Read the model definition and answer for the solid it produces. Units are mm, in the model's axes. Face numbers are marked on the shaded views. A direction names the side the tool comes from. Give positions to 0.01 mm unless a question says otherwise; leave off trailing zeros. Write each loop counter-clockwise with the first axis right and the second up, starting at its lowest first coordinate (ties: lowest second). Pieces come first, ordered by that corner, then holes. Notation, with made-up numbers: M 16,63 L 67,63 A23 cw 67,95 Z; hole C 50,12 d10. An arc over 180 degrees is marked long. Put each result on its own line as item: value.
Autodesk Inventor part; units mm, degrees
ref_plane "YZ Plane" through (0, 0, 0) normal (1, 0, 0) x (0, 1, 0)
ref_plane "XZ Plane" through (0, 0, 0) normal (0, 1, 0) x (-1, 0, 0)
ref_plane "XY Plane" through (0, 0, 0) normal (0, 0, 1) x (1, 0, 0)
sketch "Sketch_1" plane through (0, 0, 0) normal (0, 0, 1) x (1, 0, 0)
  line L0 (0, 28.85) -> (0, 9.95)
  line L1 (0, 9.95) -> (15, 9.95)
  line L2 (15, 9.95) -> (15, 28.85)
  arc A0 (15, 28.85) -> (14, 29.85) centre (14, 28.85) ccw
  line L3 (14, 29.85) -> (1, 29.85)
  arc A1 (1, 29.85) -> (0, 28.85) centre (1, 28.85) ccw
extrude "Extrusion1" add sketch "Sketch_1" against normal blind 30
sketch "Sketch_6" plane through (7.5, 0, 0) normal (1, 0, 0) x (0, 0, -1)
  line L0 (0, 21.4) -> (35, 21.4)
  line L1 (35, 21.4) -> (35, 18.15)
  line L2 (35, 18.15) -> (34.5, 18.65)
  line L3 (34.5, 18.65) -> (0.5, 18.65)
  line L4 (0.5, 18.65) -> (0, 18.15)
  line L5 (0, 18.15) -> (0, 21.4)
  line L6 (0, 21.4) -> (35, 21.4)
revolve "Revolution1" cut sketch "Sketch_6" angle 360 about axis through (7.5, 21.4, 0) along (0, 0, 1)
sketch "Sketch_4" plane through (7.5, 0, 0) normal (1, 0, 0) x (0, 0, -1)
  line L0 (0, 22.5) -> (35, 22.5)
  line L1 (35, 22.5) -> (35, 19.25)
  line L2 (35, 19.25) -> (34.5, 19.75)
  line L3 (34.5, 19.75) -> (0.5, 19.75)
  line L4 (0.5, 19.75) -> (0, 19.25)
  line L5 (0, 19.25) -> (0, 22.5)
  line L6 (0, 22.5) -> (35, 22.5)
revolve "Revolution2" cut sketch "Sketch_4" angle 360 about axis through (7.5, 22.5, 0) along (0, 0, 1)
sketch "Sketch_8" plane through (0, 21.95, 0) normal (0, 1, 0) x (1, 0, 0)
  line L0 (4.25, 0) -> (10.75, 0)
  line L1 (10.75, 0) -> (10.25, 0.5)
  line L2 (10.25, 0.5) -> (10.25, 34.5)
  line L3 (10.25, 34.5) -> (10.75, 35)
  line L4 (10.75, 35) -> (4.25, 35)
  line L5 (4.25, 35) -> (4.75, 34.5)
  line L6 (4.75, 34.5) -> (4.75, 0.5)
  line L7 (4.75, 0.5) -> (4.25, 0)
extrude "Extrusion2" cut sketch "Sketch_8" along normal mid plane 1.1
sketch "Sketch_10" plane through (0, 0, -0.5) normal (0, 0, 1) x (1, 0, 0)
  arc A0 (4.75, 21.4) -> (10.25, 21.4) centre (7.5, 21.4) ccw
  line L0 (10.25, 21.4) -> (10.25, 22.5)
  arc A1 (10.25, 22.5) -> (4.75, 22.5) centre (7.5, 22.5) ccw
  line L1 (4.75, 22.5) -> (4.75, 21.4)
extrude "Extrusion3" add sketch "Sketch_10" against normal blind 29
sketch "Sketch_11" plane through (7.5, 0, 0) normal (1, 0, 0) x (0, 0, -1)
  line L0 (0.5, 21.95) -> (29.5, 21.95)
  line L1 (29.5, 21.95) -> (29.5, 19.45)
  line L2 (29.5, 19.45) -> (29.067, 19.883)
  line L3 (29.067, 19.883) -> (0.933, 19.883)
  line L4 (0.933, 19.883) -> (0.5, 19.45)
  line L5 (0.5, 19.45) -> (0.5, 21.95)
  line L6 (0.5, 21.95) -> (29.5, 21.95)
revolve "Revolution3" cut sketch "Sketch_11" angle 360 about axis through (7.5, 21.95, -0.5) along (0, 0, 1)
thread "Thread1"
sketch "_____2" plane through (0, 9.95, 0) normal (0, 1, 0) x (1, 0, 0)
  line L0 (2.75, 17.75) -> (2.75, 14.75)
  arc A0 (2.75, 14.75) -> (7.25, 10.25) centre (7.25, 14.75) ccw
  line L1 (7.25, 10.25) -> (10.25, 10.25)
  arc A1 (10.25, 10.25) -> (12.25, 12.25) centre (10.25, 12.25) ccw
  line L2 (12.25, 12.25) -> (12.25, 15.25)
  arc A2 (12.25, 15.25) -> (7.75, 19.75) centre (7.75, 15.25) ccw
  line L3 (7.75, 19.75) -> (4.75, 19.75)
  arc A3 (4.75, 19.75) -> (2.75, 17.75) centre (4.75, 17.75) ccw
extrude "Extrusion4" add sketch "_____2" against normal blind 9.6
sketch "_____3" plane through (7.5, 0, 0) normal (1, 0, 0) x (0, 0, -1)
  line L0 (5.5, 4.65) -> (5.5, 2.35)
  arc A0 (5.5, 2.35) -> (7.5, 0.35) centre (7.5, 2.35) ccw
  line L1 (7.5, 0.35) -> (22.5, 0.35)
  arc A1 (22.5, 0.35) -> (24.5, 2.35) centre (22.5, 2.35) ccw
  line L2 (24.5, 2.35) -> (24.5, 4.65)
  line L3 (24.5, 4.65) -> (5.5, 4.65)
extrude "Extrusion5" add sketch "_____3" along normal mid plane 9.5
sketch "_____4" plane through (0, 0, -14.75) normal (0, 0, 1) x (1, 0, 0)
  line L0 (2.75, 4.25) -> (7.5, 4.65)
  line L1 (7.5, 4.65) -> (2.75, 4.65)
  line L2 (2.75, 4.65) -> (2.75, 4.25)
extrude "Extrusion6" cut sketch "_____4" along normal blind 9.5
sketch "_____5" plane through (0, 0, -15.25) normal (0, 0, 1) x (1, 0, 0)
  line L0 (7.5, 4.65) -> (12.25, 4.25)
  line L1 (12.25, 4.25) -> (12.25, 4.65)
  line L2 (12.25, 4.65) -> (7.5, 4.65)
extrude "Extrusion7" cut sketch "_____5" against normal blind 9.5
sketch "_____7" plane through (0, 0.35, 0) normal (0, 1, 0) x (1, 0, 0)
  line L0 (2.75, 17.75) -> (2.75, 14.75)
  arc A0 (2.75, 14.75) -> (7.25, 10.25) centre (7.25, 14.75) ccw
  line L1 (7.25, 10.25) -> (10.25, 10.25)
  arc A1 (10.25, 10.25) -> (12.25, 12.25) centre (10.25, 12.25) ccw
  line L2 (12.25, 12.25) -> (12.25, 15.25)
  arc A2 (12.25, 15.25) -> (7.75, 19.75) centre (7.75, 15.25) ccw
  line L3 (7.75, 19.75) -> (4.75, 19.75)
  arc A3 (4.75, 19.75) -> (2.75, 17.75) centre (4.75, 17.75) ccw
extrude "Extrusion8" add sketch "_____7" along normal blind 4.3
sketch "_____1" plane through (0, 0.35, 0) normal (0, 1, 0) x (1, 0, 0)
  line L0 (-10.5888, -9.9588) -> (25.3573, -9.9588)
  line L1 (25.3573, -9.9588) -> (25.3573, 39.1524)
  line L2 (25.3573, 39.1524) -> (-10.5888, 39.1524)
  line L3 (-10.5888, 39.1524) -> (-10.5888, -9.9588)
  arc A0 (2.75, 10.3) -> (7.55, 5.5) centre (7.55, 10.3) ccw
  line L4 (7.55, 5.5) -> (12.25, 5.5)
  line L5 (12.25, 5.5) -> (12.25, 19.7)
  arc A1 (12.25, 19.7) -> (7.45, 24.5) centre (7.45, 19.7) ccw
  line L6 (7.45, 24.5) -> (2.75, 24.5)
  line L7 (2.75, 24.5) -> (2.75, 10.3)
extrude "Extrusion9" cut sketch "_____1" along normal mid plane 19.2
sketch "Sketch_3" plane through (7.5, 0, 0) normal (1, 0, 0) x (0, 0, -1)
  line L0 (15, 0.35) -> (15, -1.45)
  line L1 (15, -1.45) -> (14.5, -1.45)
  line L2 (14.5, -1.45) -> (13, 0.35)
  line L3 (13, 0.35) -> (15, 0.35)
  line L4 (15, 0.35) -> (15, -1.45)
revolve "Revolution4" add sketch "Sketch_3" angle 360 about axis through (7.5, 0.35, -15) along (0, 1, 0)
sketch "Sketch_7" plane through (15, 0, 0) normal (1, 0, 0) x (0, 0, -1)
  line L0 (2, 15.2) -> (2, 11.95)
  line L1 (2, 11.95) -> (14, 11.95)
  line L2 (14, 11.95) -> (14, 15.2)
  line L3 (14, 15.2) -> (2, 15.2)
extrude "Extrusion10" cut sketch "Sketch_7" against normal blind 15
sketch "Sketch_5" plane through (15, 0, 0) normal (1, 0, 0) x (0, 0, -1)
  line L0 (16, 15.2) -> (16, 11.95)
  line L1 (16, 11.95) -> (28, 11.95)
  line L2 (28, 11.95) -> (28, 15.2)
  line L3 (28, 15.2) -> (16, 15.2)
extrude "Extrusion11" cut sketch "Sketch_5" against normal blind 15
sketch "Sketch_9" plane through (0, 0, 0) normal (0, 1, 0) x (-1, 0, 0)
  line L0 (0, -15.3) -> (0, -14.7)
  line L1 (0, -14.7) -> (-0.3, -15)
  line L2 (-0.3, -15) -> (0, -15.3)
extrude "Extrusion12" cut sketch "Sketch_9" along normal blind 40
sketch "Sketch_15" plane through (0, 0, 0) normal (0, 1, 0) x (-1, 0, 0)
  line L0 (-14.7, -15) -> (-15, -14.7)
  line L1 (-15, -14.7) -> (-15, -15.3)
  line L2 (-15, -15.3) -> (-14.7, -15)
extrude "Extrusion13" cut sketch "Sketch_15" along normal blind 40
sketch "Sketch_16" plane through (0, 0, 0) normal (0, 1, 0) x (-1, 0, 0)
  line L0 (-7.2, 0) -> (-7.8, 0)
  line L1 (-7.8, 0) -> (-7.5, -0.3)
  line L2 (-7.5, -0.3) -> (-7.2, 0)
extrude "Extrusion14" cut sketch "Sketch_16" along normal blind 40
sketch "Sketch_17" plane through (0, 0, 0) normal (0, 1, 0) x (-1, 0, 0)
  line L0 (-7.2, -30) -> (-7.5, -29.7)
  line L1 (-7.5, -29.7) -> (-7.8, -30)
  line L2 (-7.8, -30) -> (-7.2, -30)
extrude "Extrusion15" cut sketch "Sketch_17" along normal blind 50
properties part number "HCBRB8"
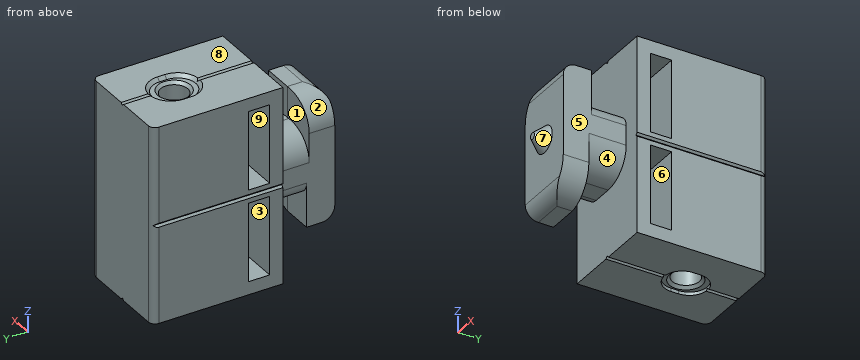
(1) Section C-C on z = -18.5 is taken. Determine the outline of the cut face in (x, y).
Result:
outline: M 0,9.95 L 2.9,9.95 L 2.9,4.65 L 2.75,4.65 L 2.75,0.35 L 12.25,0.35 L 12.25,4.25 L 10.86,4.37 L 10.86,9.95 L 15,9.95 L 15,11.95 L 0,11.95 Z; M 0,15.2 L 15,15.2 L 15,28.85 A1 ccw 14,29.85 L 1,29.85 A1 ccw 0,28.85 Z; hole C 7.5,21.95 d4.13
(2) Section A-A on y = 21.95 is taken. Determine the outline of the cut face in (x, z), and give its area (3 significant figures).
Result:
outline: M 0,-30 L 4.75,-30 L 4.75,-29.5 L 5,-29.5 L 5.43,-29.07 L 5.43,-0.93 L 5,-0.5 L 4.75,-0.5 L 4.25,0 L 0,0 L 0,-14.7 L 0.3,-15 L 0,-15.3 Z; M 9.57,-29.07 L 10,-29.5 L 10.25,-29.5 L 10.25,-30 L 15,-30 L 15,-15.3 L 14.7,-15 L 15,-14.7 L 15,0 L 10.75,0 L 10.25,-0.5 L 10,-0.5 L 9.57,-0.93 Z
area: 324 mm²
(3) Straight lines are drawn through the part: line 1 along Z through (x, y) = (3.5, 14); line 2 along X through (y, z) = (21.95, -18); line 3 along Y through (x, z) = (7.75, -8). For each, find the intervals that lie inside material, in ascending order. Write a range as from..to.
Result:
line 1: z = -30..-28, -16..-14, -2..0
line 2: x = 0..5.43, 9.57..15
line 3: y = 0.35..4.65, 9.95..11.95, 15.2..19.9, 24..29.85
(4) Given pin 1 Ø2 at (x, y) = (9, 5) entering from +Z; pin 2 Ø2 at (y, z) = (13.5, -8) entering from +X; pin 3 Ø3 at (x, y) = (7.5, 20.5) entering from +Z; pin 4 Ø6 at (x, z) = (10, -6) entering from -Y, each flat-ended and moving along its own axis, determine where each tip first touches the part or whether it passes through.
Result:
pin 1: stops at z = -5.5
pin 2: passes through
pin 3: stops at z = -0.5
pin 4: stops at y = 0.35
(5) Section B-B on z = -8.5 is taken. Determine the outline of the cut face in (x, y), and give its area (3 significant figures).
Result:
outline: M 0,9.95 L 15,9.95 L 15,11.95 L 0,11.95 Z; M 0,15.2 L 15,15.2 L 15,28.85 A1 ccw 14,29.85 L 1,29.85 A1 ccw 0,28.85 Z; M 3.1,0.35 L 12.25,0.35 L 12.25,4.65 L 7.5,4.65 L 3.1,4.28 Z; hole C 7.5,21.95 d4.13
area: 274 mm²
(6) Section D-D on z = -22 is taken. Determine the outline of the cut face in (x, y).
Result:
outline: M 0,9.95 L 15,9.95 L 15,11.95 L 0,11.95 Z; M 0,15.2 L 15,15.2 L 15,28.85 A1 ccw 14,29.85 L 1,29.85 A1 ccw 0,28.85 Z; M 2.75,0.35 L 11.66,0.35 L 11.66,4.3 L 7.5,4.65 L 2.75,4.65 Z; hole C 7.5,21.95 d4.13
(7) For a pull along Z with two mould halves and no side action, classify the marked faces 6, 7, 8 and 9 as +Z half, -Z half, draft (parallel to the pull), parting line (faces both ways), or undercut.
Result:
face 6: undercut
face 7: parting line
face 8: +Z half
face 9: undercut
(8) Which of the six approach directions +Z, -Z, +X, -X, +Y, -Y give full straight-line access (tool end or side, diameter ignored) to the marked faces 1, 2, 3, 4 and 5?
Result:
face 1: +Z, -X
face 2: +Z, -X, -Y
face 3: +X, -X
face 4: -Z, +X
face 5: +Z, -Z, +X, -Y
